from build123d import *

# Parameters (mm, degrees)
F0_W     = 22.3266
F0_H     = 22.3266
F0_W_2   = 19.7866
F0_H_2   = 19.7866
F1_DEPTH = 228.6
F2_R     = 1.905
F3_DEPTH = 22.3276
F4_R     = 1.905
F5_DEPTH = 22.3276


with BuildPart() as f1:
    # F0 (on Top) → F1 (new body)
    with BuildSketch(Plane.XY):
        Rectangle(F0_W, F0_H)
        Rectangle(F0_W_2, F0_H_2, mode=Mode.SUBTRACT)
    extrude(amount=F1_DEPTH)

    # F2 (on face) → F3 (cut, through all)
    with BuildSketch(Plane.XZ.offset(11.1633)):
        with Locations((0, 38.1)):
            Circle(F2_R)
        with Locations((0, 76.2)):
            Circle(F2_R)
        with Locations((0, 114.3)):
            Circle(F2_R)
        with Locations((0, 152.4)):
            Circle(F2_R)
        with Locations((0, 190.5)):
            Circle(F2_R)
    extrude(amount=-F3_DEPTH, mode=Mode.SUBTRACT)

    # F4 (on face) → F5 (cut, through all)
    with BuildSketch(Plane.XZ.offset(11.1633)):
        with Locations((0, 215.9)):
            Circle(F4_R)
        with Locations((7.62, 215.9)):
            Circle(F4_R)
        with Locations((0, 208.28)):
            Circle(F4_R)
    extrude(amount=-F5_DEPTH, mode=Mode.SUBTRACT)


solid = f1.part
Geometry: final body of the model. Coordinates: model frame, mm. A direction names the side the tool comes from. Round coordinates to 2 decimals unless told otherwise and drop trailing zeros. Loops run counter-clockwise (first coordinate to the right, second up) from the corner with the lowest first, then second, coordinate; pieces in that order, holes last. Notation, with made-up numbers: (47.5, 46) -> (55.5, 46) arc R12 ccw to (55.5, 68) -> close; hole circle Ø4 at (3, 78.5). An arc over 180 degrees is marked (long way). One line per question, with ' | ' between items. Start each with the question number.
1. Contact query for flat-ended pins moving along their axis: pin 1 (4.5 mm diameter, centred on x = 0, z = 38.1, fed in from -Y); pin 2 (6 mm diameter, centred on x = -4, y = -3.5, fed in from +Z). Output: stop coordinate, or through.
2. Section C-C on y = -5. Output: boundary loops of the cut face in (x, z), and give its area (3 significant figures).
3. Section A-A on z = 215.9. Output: boundary loops of the cut face in (x, y) (3 decimals).
4. Mould query, pull axis Y, two halves, no side actions, for faces 1 (the face through (-3, 11.163, 113)), 2 (the face through (-0.41, -10.54, 214.04)), 3 (the face through (9.893, 0, 113)). Classes: pulls with the +Y half, pulls with the -Y half, needs draft (parallel to the pull), parting line crosses it, or undercut.
5. Section B-B on z = 119. Output: boundary loops of the cut face in (x, y), and give its area (3 significant figures).
6. Line query: line 1 along X through (y, z) = (10.85, 215.9) (3 decimals); line 2 along Y through (x, z) = (-3, 141). Output: solid intervals per line, ascending. Write a range as [from, to].
7. Section D-D on x = 7.62. Output: boundary loops of the cut face in (y, z) (3 decimals), and give its area (3 significant figures).
8. Set-up query: faces 4 (the face through (1, 10.5, 209.9)), 5 (the face through (-2, 9.893, 113)). Return all of +Z, -Z, +X, -X, +Y, -Y with unobstructed straight access to the full face (end or side cutting, diameter ignored); none if empty.
Returned:
1) pin 1: stops at y = -11.16 | pin 2: passes through
2) outline: (-11.16, 0) -> (-9.89, 0) -> (-9.89, 228.6) -> (-11.16, 228.6) -> close; (9.89, 0) -> (11.16, 0) -> (11.16, 228.6) -> (9.89, 228.6) -> close | area: 581 mm2
3) outline: (-11.163, -11.163) -> (-1.905, -11.163) -> (-1.905, -9.893) -> (-9.893, -9.893) -> (-9.893, 9.893) -> (-1.905, 9.893) -> (-1.905, 11.163) -> (-11.163, 11.163) -> close; (1.905, -11.163) -> (5.715, -11.163) -> (5.715, -9.893) -> (1.905, -9.893) -> close; (1.905, 9.893) -> (5.715, 9.893) -> (5.715, 11.163) -> (1.905, 11.163) -> close; (9.525, -11.163) -> (11.163, -11.163) -> (11.163, 11.163) -> (9.525, 11.163) -> (9.525, 9.893) -> (9.893, 9.893) -> (9.893, -9.893) -> (9.525, -9.893) -> close
4) face 1: pulls with the +Y half | face 2: needs draft | face 3: undercut
5) outline: (-11.16, -11.16) -> (11.16, -11.16) -> (11.16, 11.16) -> (-11.16, 11.16) -> close; hole (-9.89, -9.89) -> (9.89, -9.89) -> (9.89, 9.89) -> (-9.89, 9.89) -> close | area: 107 mm2
6) line 1: x = [-11.163, -1.905], [1.905, 5.715], [9.525, 11.163] | line 2: y = [-11.16, -9.89], [9.89, 11.16]
7) outline: (-11.163, 0) -> (-9.893, 0) -> (-9.893, 213.995) -> (-11.163, 213.995) -> close; (-11.163, 217.805) -> (-9.893, 217.805) -> (-9.893, 228.6) -> (-11.163, 228.6) -> close; (9.893, 0) -> (11.163, 0) -> (11.163, 213.995) -> (9.893, 213.995) -> close; (9.893, 217.805) -> (11.163, 217.805) -> (11.163, 228.6) -> (9.893, 228.6) -> close | area: 571 mm2
8) face 4: +Y, -Y | face 5: +Z, -Z
